Build history of the part. All positions in model axes, mm. A direction names the side the tool comes from. Give positions to 0.01 mm unless a question says otherwise; leave off trailing zeros. Write each loop counter-clockwise with the first axis right and the second up, starting at its lowest first coordinate (ties: lowest second). Pieces come first, ordered by that corner, then holes.
from build123d import *

# Parameters (mm, degrees)
F2_DEPTH = 8
F4_DEPTH = 6.401
F5_SIZE  = 1.2


with BuildPart() as f2:
    # F1 (on Front) → F2 (new body, symmetric)
    with BuildSketch(Plane.XZ):
        with BuildLine():
            Line((-2.4, -4.05), (0, -4.05))
            Line((0, -4.05), (1.2, -1.65))
            Line((1.2, -1.65), (0, -1.65))
            Line((0, -1.65), (0, 0))
            Line((0, 0), (4, 0))
            ThreePointArc((4, 0), (24.3, 4.8), (44.6, 0))
            Line((44.6, 0), (48.6, 0))
            Line((48.6, 0), (48.6, -12.8))
            Line((48.6, -12.8), (50.1, -12.8))
            Line((50.1, -12.8), (50.1, -18.8))
            Line((50.1, -18.8), (52.5, -18.8))
            Line((52.5, -18.8), (52.5, 1.2))
            ThreePointArc((52.5, 1.2), (25.05, 6.4), (-2.4, 1.2))
            Line((-2.4, 1.2), (-2.4, -4.05))
        make_face()
    extrude(amount=F2_DEPTH, both=True)

    # F3 (on Top) → F4 (cut, through all)
    with BuildSketch(Plane.XY):
        Polygon((5.6, 5.6), (0, 0), (5.6, -5.6), (11.2, 0), align=None)
        Polygon((44.5, 5.6), (38.9, 0), (44.5, -5.6), (50.1, 0), align=None)
        Polygon((36.5, 0), (32.1, 4.4), (27.7, 0), (32.1, -4.4), align=None)
        Polygon((22.4, 0), (18, 4.4), (13.6, 0), (18, -4.4), align=None)
    extrude(amount=F4_DEPTH, mode=Mode.SUBTRACT)

    # F5
    f5_edges = [f2.edges().sort_by_distance(p)[0] for p in [
        (52.5, 0, -18.8),
    ]]
    chamfer(f5_edges, length=F5_SIZE)


solid = f2.part
(1) Drop flat-ended pins along their axis: pin 1 (1.5 mm diameter, centred on y = -3, z = -6, fed in from -X); pin 2 (4.5 mm diameter, centred on x = 46, y = 5.5, fed in from -Z); pin 3 (5 mm diameter, centred on x = 23, y = -5, fed in from -Z). Give the stop position or say it passes through.
(2) Probe line 1 (X direction, y = 2, z = -14.5); line 2 (X direction, y = 0.25, z = -4) (3 decimals); line 3 (Z direction, x = 25, y = 5). List the from-to ranges inside material, lowest first.
(3) Saw through at A-A, the plane z = -1. List the corners of the cut face in (x, y), plus the area to 3 significant figures.
(4) Saw through at B-B, the plane y = -6.75. List the corners of the cut face in (x, z), plus the area to 3 significant figures.
(5) Saw through at D-D, the plane y = 5. List the corners of the cut face in (x, z).
(6) Mould opens along Y. For faces 6 (the face through (49, 0, -12.8)), 7 (the face through (29.9, 2.2, 5.2)) say: +Y half, -Y half, draft (parallel to the pull), parting line (faces both ways), or undercut.
(7) Saw through at C-C, the plane x = 15. List the corners of the cut face in (y, z).
(8) 3-axis set-ups, long thin cutter, end or side, ignore diameter. For faces 1 (the face through (47.3, 2.8, 1.5)), 2 (the face through (47, 5, 0)), 3 (the face through (2, 5, 0)), 4 (the face through (41.7, -2.8, 3.1)), 5 (the face through (51.9, 0.1, -18.2)): which of +Z, -Z, +X, -X, +Y, -Y reach the whole face in a straight line?
Computed values:
1. pin 1: stops at x = 48.6
1. pin 2: stops at z = 0
1. pin 3: stops at z = 4.64
2. line 1: x = 50.1 to 52.5
2. line 2: x = -2.4 to 0.025, 48.6 to 52.5
2. line 3: z = 4.79 to 6.4
3. outline: (-2.4, -8) - (0, -8) - (0, 8) - (-2.4, 8) - close; (48.6, -8) - (52.5, -8) - (52.5, 8) - (48.6, 8) - close
3. area: 101 mm2
4. outline: (-2.4, -4.05) - (0, -4.05) - (1.2, -1.65) - (0, -1.65) - (0, 0) - (4, 0) arc R45.33 cw to (44.6, 0) - (48.6, 0) - (48.6, -12.8) - (50.1, -12.8) - (50.1, -18.8) - (51.3, -18.8) - (52.5, -17.6) - (52.5, 1.2) arc R75.05 ccw to (-2.4, 1.2) - close
4. area: 201 mm2
5. outline: (-2.4, -4.05) - (0, -4.05) - (1.2, -1.65) - (0, -1.65) - (0, 0) - (4, 0) arc R45.33 cw to (5, 0.49) - (5, 3.67) arc R75.05 ccw to (-2.4, 1.2) - close; (6.2, 1.03) arc R45.33 cw to (43.9, 0.34) - (43.9, 3.99) arc R75.05 ccw to (6.2, 3.99) - close; (45.1, 0) - (48.6, 0) - (48.6, -12.8) - (50.1, -12.8) - (50.1, -18.8) - (51.3, -18.8) - (52.5, -17.6) - (52.5, 1.2) arc R75.05 ccw to (45.1, 3.67) - close
6. face 6: draft
6. face 7: undercut
7. outline: (-8, 3.84) - (-1.4, 3.84) - (-1.4, 5.72) - (-8, 5.72) - close; (1.4, 3.84) - (8, 3.84) - (8, 5.72) - (1.4, 5.72) - close
8. face 1: +Z
8. face 2: -Z, +Y, -Y
8. face 3: +Y, -Y
8. face 4: +Z, -Z
8. face 5: -Z, +X, +Y, -Y
